The listing builds one solid part. Answer for the finished solid, in the listing's coordinates (mm). Face numbers are marked on the shaded views. A direction names the side the tool comes from. Round coordinates to 2 decimals unless told otherwise and drop trailing zeros. Write each loop counter-clockwise with the first axis right and the second up, starting at its lowest first coordinate (ties: lowest second). Pieces come first, ordered by that corner, then holes. Notation, with made-up numbers: (-1.5, 62) - (49.5, 62) arc R15 ccw to (49.5, 67) - close; hole circle Ø9 at (38.5, 53.25). An arc over 180 degrees is marked (long way). Use a Markdown table: item, result. Add a question column.
1) A tool of negligible diameter and unlimited length cuts with its end or side. For the marked faces 4, 5 and 6, from which of +Z, -Z, +X, -X, +Y, -Y can it reach the whole face along a straight path? Write none if from no direction.
2) Each of these flat-tipped pins is pushed along its axis until it touches: P1, Ø4, axis at y = -1, z = 30, coming from the -X side; P2, Ø4, axis at y = -0.5, z = 11.5, coming from the +X side; P3, Ø1, axis at x = 1, z = 41.5, coming from the +Y side; P4, Ø1, axis at y = -3, z = 45, coming from the +X side. Where does it stop, or does it pass through?
3) Find the intervals of material crossed by probe 1 along Y at (x, z) = (1.5, 49); probe 2 along Z at (x, y) = (-8, 3.5); probe 3 along Z at (x, y) = (-1.25, 2), in increasing order. Write a range as from..to.
4) Determine the mould class of the marked faces 1, 2 and 3 for opening direction X: +X half, -X half, draft (parallel to the pull), parting line (faces both ways), or undercut.
5) A cutting plane is placed at B-B (z = 10). Give the vertices of the cut face in (x, y), then the cut area to 4 significant figures.
6) A cutting plane is placed at A-A (y = -2.75). Give the vertices of the cut face in (x, z).
7) A cutting plane is placed at D-D (x = -5.5). Give the vertices of the cut face in (y, z).
8) A cutting plane is placed at C-C (z = 17). Give the vertices of the cut face in (x, y).
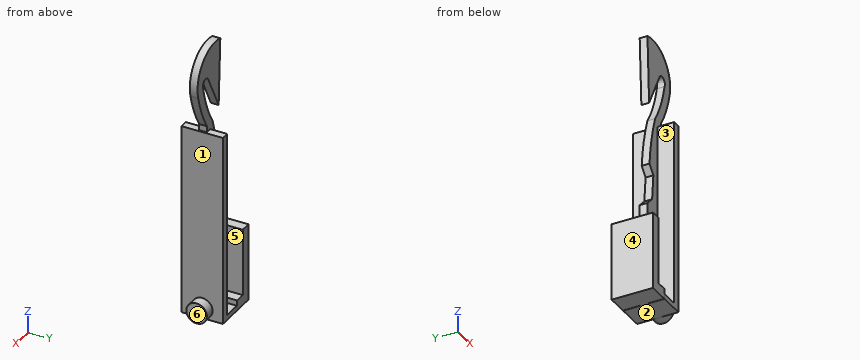
```python
from build123d import *

# Parameters (mm, degrees)
PAD003_DEPTH = 4
SKETCH002_R  = 2
PAD004_DEPTH = 2
PAD005_DEPTH = 4
PAD_DEPTH    = 0.75


with BuildPart() as pad003:
    # Sketch003 → Pad003 (new body, symmetric)
    with BuildSketch(Plane.XZ):
        Polygon((-9, 15), (-7, 15), (-7, 2), (-5, 2), (-5, 0), (-9, 0), align=None)
    extrude(amount=PAD003_DEPTH, both=True)


with BuildPart() as pad004:
    # Sketch002 → Pad004 (new body)
    with BuildSketch(Plane.YZ):
        with Locations((0, 2)):
            Circle(SKETCH002_R)
    extrude(amount=PAD004_DEPTH)


with BuildPart() as pad005:
    # Sketch → Pad005 (new body, symmetric)
    with BuildSketch(Plane.XZ):
        Polygon((-1.5, 37), (0, 37), (0, 0), (-4.908648, 0), (-4.908648, 1), (-1.5, 1), align=None)
    extrude(amount=PAD005_DEPTH, both=True)


with BuildPart() as fusion:
    # Sketch001 → Pad (new body, symmetric)
    with BuildSketch(Plane.XZ):
        with BuildLine():
            Line((0, 0), (0, 28.218657))
            ThreePointArc((-0.280961, 38.218657), (-0.265608, 33.215142), (0, 28.218657))
            ThreePointArc((-0.280961, 38.218657), (1.567466, 41.71926), (2.817294, 45.475433))
            ThreePointArc((2.817294, 45.475433), (1.179618, 51.6371), (-5, 53.205675))
            Line((-4.419163, 40.218657), (-5, 53.205675))
            Line((-4.419163, 40.218657), (-0.732708, 47.318661))
            ThreePointArc((1.042293, 46.397047), (0.615603, 47.745362), (-0.732708, 47.318661))
            ThreePointArc((-2.280961, 38.218657), (-0.238148, 42.152959), (1.042293, 46.397047))
            ThreePointArc((-2.280961, 38.218657), (-3.600955, 33.282656), (-4.280961, 28.218657))
            Line((-4.280961, 28.218657), (-2.922591, 26.599815))
            Line((-3.35837, 21.618842), (-2.922591, 26.599815))
            Line((-5, 20), (-3.35837, 21.618842))
            Line((-5, 0), (-5, 20))
            Line((0, 0), (-5, 0))
        make_face()
    extrude(amount=PAD_DEPTH, both=True)

    # Fusion: union Pad003, Pad004, Pad005
    add(pad003.part)
    add(pad004.part)
    add(pad005.part)


solid = fusion.part
```
Entries:
| question | item | result |
|---|---|---|
| 1 | face 4 | +Z, -Z, -X, +Y, -Y |
| 1 | face 5 | +Z, +Y, -Y |
| 1 | face 6 | -Z, +X, +Y, -Y |
| 2 | P1 | stops at x = -4.28 |
| 2 | P2 | stops at x = 0 |
| 2 | P3 | stops at y = 0.75 |
| 2 | P4 | passes through |
| 3 | probe 1 | y = -0.75..0.75 |
| 3 | probe 2 | z = 0..15 |
| 3 | probe 3 | z = 0..37 |
| 4 | face 1 | +X half |
| 4 | face 2 | draft |
| 4 | face 3 | undercut |
| 5 | outline | (-9, -4) - (-7, -4) - (-7, 4) - (-9, 4) - close; (-5, -0.75) - (-1.5, -0.75) - (-1.5, -4) - (0, -4) - (0, 4) - (-1.5, 4) - (-1.5, 0.75) - (-5, 0.75) - close |
| 5 | area | 33.25 mm² |
| 6 | outline | (-9, 0) - (-5, 0) - (-5, 2) - (-7, 2) - (-7, 15) - (-9, 15) - close; (-4.91, 0) - (0, 0) - (0, 37) - (-1.5, 37) - (-1.5, 1) - (-4.91, 1) - close |
| 7 | outline | (-4, 0) - (4, 0) - (4, 2) - (-4, 2) - close |
| 8 | outline | (-5, -0.75) - (-1.5, -0.75) - (-1.5, -4) - (0, -4) - (0, 4) - (-1.5, 4) - (-1.5, 0.75) - (-5, 0.75) - close |
